```python
from build123d import *

# Parameters (mm, degrees)
SKETCH1_W           = 27
SKETCH1_H           = 30
SKETCH1_W_2         = 22
SKETCH1_H_2         = 25
BOSS_EXTRUDE1_DEPTH = 28
SKETCH2_R           = 2.5
CUT_EXTRUDE1_DEPTH  = 14
SKETCH3_W           = 5
SKETCH3_H           = 4.2
CUT_EXTRUDE2_DEPTH  = 14
SKETCH4_R           = 4.75
CUT_EXTRUDE3_DEPTH  = 58
SKETCH5_W           = 27
SKETCH5_H           = 30
BOSS_EXTRUDE2_DEPTH = 2
SKETCH6_W           = 27
SKETCH6_H           = 32.4
BOSS_EXTRUDE3_DEPTH = 2
SKETCH7_R           = 1.7
BOSS_EXTRUDE4_DEPTH = 3
FILLET11_R          = 5


with BuildPart() as part:
    # Sketch1 → Boss-Extrude1 (new body)
    with BuildSketch(Plane.XY):
        with Locations((0, 1.2)):
            Rectangle(SKETCH1_W, SKETCH1_H)
        with Locations((0, 1.108503026)):
            Rectangle(SKETCH1_W_2, SKETCH1_H_2, mode=Mode.SUBTRACT)
    extrude(amount=BOSS_EXTRUDE1_DEPTH)

    # Sketch2 → Cut-Extrude1 (cut, symmetric)
    with BuildSketch(Plane.ZY.offset(13.5)):
        with Locations(Location((17, 1.2, 0), (0, 0, 180))):
            Circle(SKETCH2_R)
    extrude(amount=CUT_EXTRUDE1_DEPTH, both=True, mode=Mode.SUBTRACT)

    # Sketch3 → Cut-Extrude2 (cut, symmetric)
    with BuildSketch(Plane(origin=(13.5, 0, 0), x_dir=(0, 0, -1), z_dir=(1, 0, 0))):
        with Locations((-17, 1.2)):
            Rectangle(SKETCH3_W, SKETCH3_H)
    extrude(amount=CUT_EXTRUDE2_DEPTH, both=True, mode=Mode.SUBTRACT)

    # Sketch4 → Cut-Extrude3 (cut)
    with BuildSketch(Plane.XZ.offset(13.8)):
        with Locations(Location((0, 14, 0), (0, 0, 270))):
            Circle(SKETCH4_R)
    extrude(amount=-CUT_EXTRUDE3_DEPTH, mode=Mode.SUBTRACT)

    # Sketch5 → Boss-Extrude2 (add)
    with BuildSketch(Plane.XY.offset(28)):
        with Locations((0, 1.2)):
            Rectangle(SKETCH5_W, SKETCH5_H)
    extrude(amount=BOSS_EXTRUDE2_DEPTH)

    # Sketch6 → Boss-Extrude3 (add)
    with BuildSketch(Plane(origin=(0, 0, 0), x_dir=(-1, 0, 0), z_dir=(0, 0, -1))):
        Rectangle(SKETCH6_W, SKETCH6_H)
    extrude(amount=BOSS_EXTRUDE3_DEPTH)

    # Sketch7 → Boss-Extrude4 (add)
    with BuildSketch(Plane(origin=(0, 0, -2), x_dir=(-1, 0, 0), z_dir=(0, 0, -1))):
        Polygon((-13.5, 0), (-13.5, 3), (-19.5, 3), (-19.5, -3), (-13.5, -3), align=None)
        with Locations((-16.5, 0)):
            Circle(SKETCH7_R, mode=Mode.SUBTRACT)
    boss_extrude4 = extrude(amount=-BOSS_EXTRUDE4_DEPTH)

    # Mirror2: Boss-Extrude4 across plane
    add(boss_extrude4.mirror(Plane(origin=(0, 0, 0), x_dir=(0, 0, 1), z_dir=(1, 0, 0))))

    # Fillet11
    fillet11_edges = [part.edges().sort_by_distance(p)[0] for p in [
        (-13.5, 1.2, 30),
        (13.5, 1.2, 30),
    ]]
    fillet(fillet11_edges, radius=FILLET11_R)

    # Mirror1: Boss-Extrude4 across plane
    add(boss_extrude4.mirror(Plane(origin=(0, 0, 0), x_dir=(0, 0, 1), z_dir=(1, 0, 0))))


solid = part.part
```
The listing builds one solid part. Answer for the finished solid, in the listing's coordinates (mm). A direction names the side the tool comes from. Coordinates: 2 decimals unless noted, no trailing zeros. Order: outer loops, then holes, each group sorted by start corner. A loop starts at its lowest first (then second) coordinate and runs counter-clockwise, first axis right, second up. Notation, with made-up numbers: M 28,-1.75 L 84,-1.75 A16 cw 84,26.25 Z; hole C 50.5,89 d8. An arc over 180 degrees is marked long. Answer as a JSON object with one key per item and string values. Group by question number.
1. Straight lines are drawn through the part: line 1 (X direction, y = 13, z = 20); line 2 (Y direction, x = 4.5, z = 23); line 3 (Z direction, x = 7, y = -11). For each, find the intervals that lie inside material, in ascending order.
2. Determine the mould class of faces 1 (the flat face through (-5, 13.609, 14)), 2 (the cylindrical face through (14.88, 0.51, -0.52)), 3 (the flat face through (-15.2, 1.4, 1)) for opening direction Z: released by +Z, released by -Z, zero draft, split by the parting line, or undercut.
3. A tool of negligible diameter and unlimited length cuts with its end or side. For faces 4 (the flat face through (12, -0.9, 17)), 5 (the flat face through (17, -3, -1)), 6 (the flat face through (-3, -13.8, 18)), 7 (the flat face through (-17, -3, -1)), 8 (the flat face through (0, 1, 28)), from which of +Z, -Z, +X, -X, +Y, -Y can it reach the whole face along a straight path? Write none if from no direction.
4. Section C-C on z = 14 is taken. Write down the section's boundary in (x, y), then the cut area to 4 significant figures.
5. Flat-ended cylindrical pins translate along their axes: P1, Ø2.5, axis at x = 16.5, y = 0, coming from the -Z side; P2, Ø1.8, axis at x = 15.5, y = -0.5, coming from the +Z side; P3, Ø11, axis at x = -3.5, z = 16.5, coming from the -Y side; P4, Ø0.8, axis at x = 12.5, y = 0, coming from the +Z side. Find the tip coordinate at first contact, or state that the pin passes through.
6. Section B-B on y = 13 is taken. Write down the section's boundary in (x, z).
7. Section A-A on x = 16.5 is taken. Write down the section's boundary in (y, z), then the cut area to 3 significant figures.
8. Section D-D on x = 5.5 is taken. Write down the section's boundary in (y, z).
Values follow:
{
 "1": {"line 1": "-13.5 to -11, 11 to 13.5", "line 2": "-13.8 to -11.39, 13.61 to 16.2", "line 3": "-2 to 0, 28 to 30"},
 "2": {"face 1": "undercut", "face 2": "zero draft", "face 3": "released by +Z"},
 "3": {"face 4": "+X", "face 5": "+Z, -Z, +X, -Y", "face 6": "+Z, +X, -X, -Y", "face 7": "+Z, -Z, -X, -Y", "face 8": "none"},
 "4": {"outline": "M -13.5,-13.8 L -4.75,-13.8 L -4.75,-11.39 L -11,-11.39 L -11,13.61 L -4.75,13.61 L -4.75,16.2 L -13.5,16.2 Z; M 4.75,-13.8 L 13.5,-13.8 L 13.5,16.2 L 4.75,16.2 L 4.75,13.61 L 11,13.61 L 11,-11.39 L 4.75,-11.39 Z", "area": "212.5 mm2"},
 "5": {"P1": "through", "P2": "z = 1", "P3": "y = -13.8", "P4": "z = 28.47"},
 "6": {"outline": "M -13.5,-2 L 13.5,-2 L 13.5,25 A5 ccw 8.5,30 L -8.5,30 A5 ccw -13.5,25 Z; hole M -11,0 L 11,0 L 11,28 L -11,28 Z"},
 "7": {"outline": "M -3,-2 L -1.7,-2 L -1.7,1 L -3,1 Z; M 1.7,-2 L 3,-2 L 3,1 L 1.7,1 Z", "area": "7.80 mm2"},
 "8": {"outline": "M -16.2,-2 L 16.2,-2 L 16.2,30 L -13.8,30 L -13.8,0 L -16.2,0 Z; hole M -11.39,0 L 13.61,0 L 13.61,28 L -11.39,28 Z"}
}
